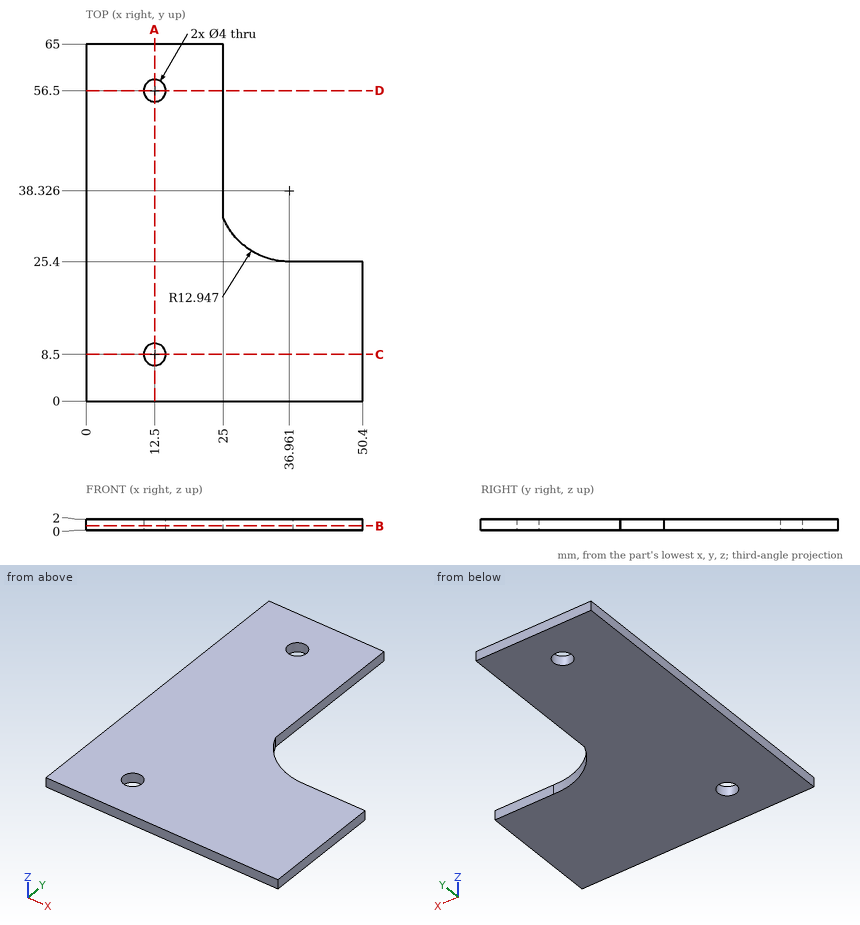
Geometry check sheet. Reference: drawing and pictorial views, mm from the part's lowest x, y, z. Coordinates: 2 decimals unless noted, no trailing zeros. Loops run counter-clockwise (first coordinate to the right, second up) from the corner with the lowest first, then second, coordinate; pieces in that order, holes last. Notation, with made-up numbers: (35, -19.75) - (54, -19.75) arc R21 ccw to (54, -13.75) - close; hole circle Ø6 at (69, -29.5). An arc over 180 degrees is marked (long way). Return JSON: item names as keys, results as strings.
1. Thickness scan on L1, parallel to Y at x = 12.5, z = 1.15; L2, parallel to Y at x = 11.5, z = 1.6; L3, parallel to X at y = 52.5, z = 0.35. Record the ranges inside material, lowest first.
Established:
{"L1": "y = 0 to 6.5, 10.5 to 54.5, 58.5 to 65", "L2": "y = 0 to 6.77, 10.23 to 54.77, 58.23 to 65", "L3": "x = 0 to 25"}
2. Section check A-A, the plane x = 12.5. Record the boundary of the cut face in (y, z).
Established:
{"outline": "(0, 0) - (6.5, 0) - (6.5, 2) - (0, 2) - close; (10.5, 0) - (54.5, 0) - (54.5, 2) - (10.5, 2) - close; (58.5, 0) - (65, 0) - (65, 2) - (58.5, 2) - close"}
3. Go/stop test with a flat-tipped pin: pin 1 (3.5 mm diameter, centred on x = 12.5, y = 8.5, fed in from -Z). Record where the tip stops, or that it passes through.
Established:
{"pin 1": "passes through"}
4. Section check C-C, the plane y = 8.5. Record the boundary of the cut face in (x, z).
Established:
{"outline": "(0, 0) - (10.5, 0) - (10.5, 2) - (0, 2) - close; (14.5, 0) - (50.4, 0) - (50.4, 2) - (14.5, 2) - close"}
5. Section check D-D, the plane y = 56.5. Record the boundary of the cut face in (x, z).
Established:
{"outline": "(0, 0) - (10.5, 0) - (10.5, 2) - (0, 2) - close; (14.5, 0) - (25, 0) - (25, 2) - (14.5, 2) - close"}
6. Section check B-B, the plane z = 0.75. Record the boundary of the cut face in (x, y) (1 decimal), then the cut area to 3 significant figures.
Established:
{"outline": "(0, 0) - (50.4, 0) - (50.4, 25.4) - (37.7, 25.4) arc R12.9 cw to (25, 33.4) - (25, 65) - (0, 65) - close; hole circle Ø4 at (12.5, 8.5); hole circle Ø4 at (12.5, 56.5)", "area": "2,270 mm2"}
